Build history of the part. All positions in model axes, mm. Round coordinates to 2 decimals unless told otherwise and drop trailing zeros. Write each loop counter-clockwise with the first axis right and the second up, starting at its lowest first coordinate (ties: lowest second). Pieces come first, ordered by that corner, then holes.
1) Wall check: probe 1 along Y at (x, z) = (-57.15, 0.25); probe 2 along Y at (x, z) = (-56, 0.5); probe 3 along Y at (x, z) = (-19.05, -1). Give the ranges that are in metal, low to high.
2) Saw through at D-D (y = -57.15). Write the cut outline in (x, z) (3 decimals), plus the area to 3 significant figures.
3) Flat gauge pins, fed straight in: pin 1 (13.5 mm diameter, centred on x = -57.15, y = -19.05, fed in from -Z) (3 decimals); pin 2 (5 mm diameter, centred on x = 19.05, y = -57.15, fed in from +Z); pin 3 (1.5 mm diameter, centred on x = 7, z = -2.5, fed in from +Y); pin 4 (1.5 mm diameter, centred on x = -32.5, z = -1.5, fed in from +Y). Where does each tip first touch, or does it go through?
4) Saw through at A-A (y = -19.05). Write the cut outline in (x, z) (3 decimals).
5) Saw through at B-B (x = 19.05). Write the cut outline in (y, z) (3 decimals).
6) Saw through at C-C (z = -2). Write the cut outline in (x, y).
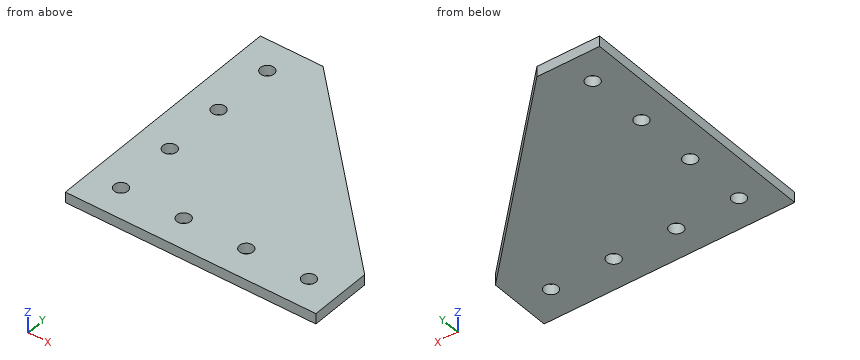
from build123d import *

# Parameters (mm, degrees)
BOSS_EXTRUDE1_DEPTH      = 3.175
BOSS_EXTRUDE1_DEPTH_BACK = 3.175
SKETCH4_R                = 4.1656
CUT_EXTRUDE1_DEPTH       = 7.35


with BuildPart() as part:
    # Sketch3 → Boss-Extrude1 (new body, two sides)
    with BuildSketch(Plane.XY) as boss_extrude1_sk:
        Polygon((76.2, -38.1), (76.2, -76.2), (-76.2, -76.2), (-76.2, 76.2), (-38.1, 76.2), align=None)
    extrude(amount=BOSS_EXTRUDE1_DEPTH)
    extrude(boss_extrude1_sk.sketch, amount=-BOSS_EXTRUDE1_DEPTH_BACK)

    # Sketch4 → Cut-Extrude1 (cut, through all)
    with BuildSketch(Plane.XY.offset(3.175)):
        with Locations((-57.15, -57.15)):
            Circle(SKETCH4_R)
        with Locations((-19.05, -57.15)):
            Circle(SKETCH4_R)
        with Locations((19.05, -57.15)):
            Circle(SKETCH4_R)
        with Locations((-57.15, -19.05)):
            Circle(SKETCH4_R)
        with Locations((-57.15, 19.05)):
            Circle(SKETCH4_R)
        with Locations((57.15, -57.15)):
            Circle(SKETCH4_R)
        with Locations((-57.15, 57.15)):
            Circle(SKETCH4_R)
    extrude(amount=-CUT_EXTRUDE1_DEPTH, mode=Mode.SUBTRACT)


solid = part.part
Evaluation:
1. probe 1: y = -76.2 to -61.32, -52.98 to -23.22, -14.88 to 14.88, 23.22 to 52.98, 61.32 to 76.2
1. probe 2: y = -76.2 to -61.15, -53.15 to -23.05, -15.05 to 15.05, 23.05 to 53.15, 61.15 to 76.2
1. probe 3: y = -76.2 to -61.32, -52.98 to 57.15
2. outline: (-76.2, -3.175) - (-61.316, -3.175) - (-61.316, 3.175) - (-76.2, 3.175) - close; (-52.984, -3.175) - (-23.216, -3.175) - (-23.216, 3.175) - (-52.984, 3.175) - close; (-14.884, -3.175) - (14.884, -3.175) - (14.884, 3.175) - (-14.884, 3.175) - close; (23.216, -3.175) - (52.984, -3.175) - (52.984, 3.175) - (23.216, 3.175) - close; (61.316, -3.175) - (76.2, -3.175) - (76.2, 3.175) - (61.316, 3.175) - close
2. area: 756 mm2
3. pin 1: stops at z = -3.175
3. pin 2: passes through
3. pin 3: stops at y = 31.85
3. pin 4: stops at y = 71.35
4. outline: (-76.2, -3.175) - (-61.316, -3.175) - (-61.316, 3.175) - (-76.2, 3.175) - close; (-52.984, -3.175) - (57.15, -3.175) - (57.15, 3.175) - (-52.984, 3.175) - close
5. outline: (-76.2, -3.175) - (-61.316, -3.175) - (-61.316, 3.175) - (-76.2, 3.175) - close; (-52.984, -3.175) - (19.05, -3.175) - (19.05, 3.175) - (-52.984, 3.175) - close
6. outline: (-76.2, -76.2) - (76.2, -76.2) - (76.2, -38.1) - (-38.1, 76.2) - (-76.2, 76.2) - close; hole circle Ø8.33 at (-57.15, -57.15); hole circle Ø8.33 at (-57.15, -19.05); hole circle Ø8.33 at (-57.15, 19.05); hole circle Ø8.33 at (-57.15, 57.15); hole circle Ø8.33 at (-19.05, -57.15); hole circle Ø8.33 at (19.05, -57.15); hole circle Ø8.33 at (57.15, -57.15)
